from build123d import *

# Parameters (mm, degrees)
EXTRUDE_1_DEPTH     = 30
CUT_EXTRUDE_1_DEPTH = 84.666002653
SKETCH_4_R          = 5
CUT_EXTRUDE_2_DEPTH = 84.666002653


with BuildPart() as part:
    # Эскиз1 → Бобышка-Вытянуть1 (new body)
    with BuildSketch(Plane.XY):
        with BuildLine():
            Line((60, -50), (60, -40))
            ThreePointArc((60, -40), (50, -38.729833462), (40.635083269, -35))
            Line((40.635083269, -35), (25, -35))
            Line((25, -35), (25, -50))
            Line((25, -50), (60, -50))
        make_face()
        with BuildLine():
            Line((25, -35), (40.635083269, -35))
            ThreePointArc((40.635083269, -35), (31.715728753, -28.284271247), (25, -19.364916731))
            Line((25, -19.364916731), (25, -35))
        make_face()
        with BuildLine():
            Line((25, 19.364916731), (25, 35))
            Line((25, 35), (-60, 35))
            Line((-60, 35), (-60, -35))
            Line((-60, -35), (25, -35))
            Line((25, -35), (25, -19.364916731))
            ThreePointArc((25, -19.364916731), (20, 0), (25, 19.364916731))
        make_face()
        with BuildLine():
            ThreePointArc((25, 19.364916731), (31.715728753, 28.284271247), (40.635083269, 35))
            Line((40.635083269, 35), (25, 35))
            Line((25, 35), (25, 19.364916731))
        make_face()
        with BuildLine():
            ThreePointArc((40.635083269, 35), (50, 38.729833462), (60, 40))
            Line((60, 40), (60, 50))
            Line((60, 50), (25, 50))
            Line((25, 50), (25, 35))
            Line((25, 35), (40.635083269, 35))
        make_face()
    extrude(amount=EXTRUDE_1_DEPTH)

    # Эскиз3 → Вырез-Вытянуть1 (cut, through all)
    with BuildSketch(Plane.XY.offset(30)):
        with BuildLine():
            Line((-46.5, 25.5), (6.5, 25.5))
            ThreePointArc((6.5, 25.5), (15, 17), (6.5, 8.5))
            Line((6.5, 8.5), (-46.5, 8.5))
            ThreePointArc((-46.5, 8.5), (-55, 17), (-46.5, 25.5))
        make_face()
        with BuildLine():
            Line((-46.5, -25.5), (6.5, -25.5))
            ThreePointArc((6.5, -25.5), (15, -17), (6.5, -8.5))
            Line((6.5, -8.5), (-46.5, -8.5))
            ThreePointArc((-46.5, -8.5), (-55, -17), (-46.5, -25.5))
        make_face()
    extrude(amount=-CUT_EXTRUDE_1_DEPTH, mode=Mode.SUBTRACT)

    # Эскиз4 → Вырез-Вытянуть2 (cut, through all)
    with BuildSketch(Plane.XY.offset(30)):
        with Locations((-38, 0)):
            Circle(SKETCH_4_R)
    extrude(amount=-CUT_EXTRUDE_2_DEPTH, mode=Mode.SUBTRACT)


solid = part.part
Read the model definition and answer for the solid it produces. Units are mm, in the model's axes. A direction names the side the tool comes from. Give positions to 0.01 mm unless a question says otherwise; leave off trailing zeros. Write each loop counter-clockwise with the first axis right and the second up, starting at its lowest first coordinate (ties: lowest second). Pieces come first, ordered by that corner, then holes. Notation, with made-up numbers: M 57.5,42.25 L 87.5,42.25 A20 ccw 87.5,79.25 Z; hole C 7,9.25 d9. An arc over 180 degrees is marked long. One line per item, written item: value. Start each with the question number.
(1) Find section B-B (y = 0). Determine the outline of the cut face in (x, z), plus the area to 3 significant figures.
(2) Determine the mould class of faces 1 (the flat face through (-17, 35, 15)), 2 (the cylindrical face through (-55, 17, 15)), 3 (the flat face through (25, 43, 15)), 4 (the flat face through (-20, -25.5, 15)) for opening direction Y: pulls with the +Y half, pulls with the -Y half, needs draft (parallel to the pull), parting line crosses it, or undercut.
(3) Find section A-A (x = -35). Determine the outline of the cut face in (y, z).
(4) Find the intervals of material crossed by line 1 (Y direction, x = -38, z = 10.25); line 2 (Y direction, x = -10.5, z = 6.5); line 3 (Y direction, x = -49.5, z = 22.25), in increasing order.
(5) Find section D-D (x = 31). Determine the outline of the cut face in (y, z).
(6) A tool of negligible diameter and unlimited length cuts with its end or side. For faces 5 (the flat face through (25, -42, 15)), 6 (the flat face through (-1, 1, 30)), 7 (the cylindrical face through (15, 17, 15)), from which of +Z, -Z, +X, -X, +Y, -Y can it reach the whole face along a straight path? Write none if from no direction.
(7) Flat-ended cylindrical pins translate along their axes: pin 1 Ø15 at (x, z) = (1.5, 21.5) entering from +Y; pin 2 Ø12 at (x, z) = (-3.5, 15.5) entering from -Y; pin 3 Ø7.5 at (y, z) = (-46, 11) entering from -X; pin 4 Ø6 at (x, y) = (-38, 0) entering from -Z. Find the tip coordinate at first contact, or state that the pin passes through.
(8) Find section C-C (z = 6.25). Determine the outline of the cut face in (x, y), plus the area to 3 significant figures.
Results below:
1. outline: M -60,0 L -43,0 L -43,30 L -60,30 Z; M -33,0 L 20,0 L 20,30 L -33,30 Z
1. area: 2,100 mm^2
2. face 1: pulls with the +Y half
2. face 2: undercut
2. face 3: needs draft
2. face 4: undercut
3. outline: M -35,0 L -25.5,0 L -25.5,30 L -35,30 Z; M -8.5,0 L -4,0 L -4,30 L -8.5,30 Z; M 4,0 L 8.5,0 L 8.5,30 L 4,30 Z; M 25.5,0 L 35,0 L 35,30 L 25.5,30 Z
4. line 1: y = -35 to -25.5, -8.5 to -5, 5 to 8.5, 25.5 to 35
4. line 2: y = -35 to -25.5, -8.5 to 8.5, 25.5 to 35
4. line 3: y = -35 to -24.95, -9.05 to 9.05, 24.95 to 35
5. outline: M -50,0 L -27.55,0 L -27.55,30 L -50,30 Z; M 27.55,0 L 50,0 L 50,30 L 27.55,30 Z
6. face 5: +Z, -Z, -X, -Y
6. face 6: +Z, +X, -X, +Y, -Y
6. face 7: +Z, -Z
7. pin 1: stops at y = 35
7. pin 2: stops at y = -35
7. pin 3: stops at x = 25
7. pin 4: passes through
8. outline: M -60,-35 L 25,-35 L 25,-50 L 60,-50 L 60,-40 A40 cw 60,40 L 60,50 L 25,50 L 25,35 L -60,35 Z; hole M -46.5,-25.5 L 6.5,-25.5 A8.5 ccw 6.5,-8.5 L -46.5,-8.5 A8.5 ccw Z; hole M -46.5,8.5 L 6.5,8.5 A8.5 ccw 6.5,25.5 L -46.5,25.5 A8.5 ccw Z; hole C -38,0 d10
8. area: 4,600 mm^2
